```python
from build123d import *

# Parameters (mm, degrees)
SKETCH1_R           = 28
SKETCH1_R_2         = 19.25
BOSS_EXTRUDE1_DEPTH = 2
SKETCH2_R           = 22.15
SKETCH2_R_2         = 19.25
BOSS_EXTRUDE2_DEPTH = 1
SKETCH3_R           = 1.375
CUT_EXTRUDE1_DEPTH  = 4
SKETCH4_W           = 12.894615696
SKETCH4_H           = 54.223512158
CUT_EXTRUDE2_DEPTH  = 4
FILLET1_R           = 10
SKETCH5_R           = 2.35
CUT_EXTRUDE3_DEPTH  = 1.5
CHAMFER2_SIZE       = 0.9
CHAMFER1_SIZE       = 1
CHAMFER3_SIZE       = 1.25


with BuildPart() as part:
    # Sketch1 → Boss-Extrude1 (new body)
    with BuildSketch(Plane.XY):
        Circle(SKETCH1_R)
        Circle(SKETCH1_R_2, mode=Mode.SUBTRACT)
    extrude(amount=BOSS_EXTRUDE1_DEPTH)

    # Sketch2 → Boss-Extrude2 (add)
    with BuildSketch(Plane(origin=(0, 0, 0), x_dir=(-1, 0, 0), z_dir=(0, 0, -1))):
        Circle(SKETCH2_R)
        Circle(SKETCH2_R_2, mode=Mode.SUBTRACT)
    extrude(amount=BOSS_EXTRUDE2_DEPTH)

    # Sketch3 → Cut-Extrude1 (cut, through all)
    with BuildSketch(Plane.XY.offset(2)):
        with Locations((0, 23.75)):
            Circle(SKETCH3_R)
        with Locations((20.56810334, 11.875)):
            Circle(SKETCH3_R)
        with Locations((20.56810334, -11.875)):
            Circle(SKETCH3_R)
        with Locations((0, -23.75)):
            Circle(SKETCH3_R)
        with Locations((-20.56810334, -11.875)):
            Circle(SKETCH3_R)
        with Locations((-20.56810334, 11.875)):
            Circle(SKETCH3_R)
    extrude(amount=-CUT_EXTRUDE1_DEPTH, mode=Mode.SUBTRACT)

    # Sketch4 → Cut-Extrude2 (cut, through all)
    with BuildSketch(Plane.XY.offset(2)):
        with Locations((30.947307848, -0.328141479)):
            Rectangle(SKETCH4_W, SKETCH4_H)
        with Locations((-30.947307848, -0.328141479)):
            Rectangle(SKETCH4_W, SKETCH4_H)
    extrude(amount=-CUT_EXTRUDE2_DEPTH, mode=Mode.SUBTRACT)

    # Fillet1
    fillet1_edges = [part.edges().sort_by_distance(p)[0] for p in [
        (24.5, -13.555441712, 1),
        (24.5, 13.555441712, 1),
        (-24.5, 13.555441712, 1),
        (-24.5, -13.555441712, 1),
    ]]
    fillet(fillet1_edges, radius=FILLET1_R)

    # Sketch5 → Cut-Extrude3 (cut)
    with BuildSketch(Plane.XY.offset(2)):
        with Locations((0, 23.75)):
            Circle(SKETCH5_R)
        with Locations((20.56810334, 11.875)):
            Circle(SKETCH5_R)
        with Locations((-20.56810334, 11.875)):
            Circle(SKETCH5_R)
        with Locations((20.56810334, -11.875)):
            Circle(SKETCH5_R)
        with Locations((0, -23.75)):
            Circle(SKETCH5_R)
        with Locations((-20.56810334, -11.875)):
            Circle(SKETCH5_R)
    extrude(amount=-CUT_EXTRUDE3_DEPTH, mode=Mode.SUBTRACT)

    # Chamfer2
    chamfer2_edges = [part.edges().sort_by_distance(p)[0] for p in [
        (-2.35, 23.75, 0.5),
        (-22.91810334, -11.875, 0.5),
        (-2.35, -23.75, 0.5),
        (18.21810334, -11.875, 0.5),
        (-22.91810334, 11.875, 0.5),
        (18.21810334, 11.875, 0.5),
    ]]
    chamfer(chamfer2_edges, length=CHAMFER2_SIZE)

    # Chamfer1
    chamfer1_edges = [part.edges().sort_by_distance(p)[0] for p in [
        (-19.25, 0, 2),
        (0, 28, 2),
        (24.5, 0, 2),
        (-24.5, 0, 2),
        (0, -28, 2),
        (-24.001461876, 13.783412326, 2),
        (-24.001461876, -13.783412326, 2),
        (24.001461876, -13.783412326, 2),
        (24.001461876, 13.783412326, 2),
    ]]
    chamfer(chamfer1_edges, length=CHAMFER1_SIZE)

    # Chamfer3
    chamfer3_edges = [part.edges().sort_by_distance(p)[0] for p in [
        (19.25, 0, -1),
    ]]
    chamfer(chamfer3_edges, length=CHAMFER3_SIZE)


solid = part.part
```
Work out the finished part from the listing and answer in its coordinate system (mm). A direction names the side the tool comes from. Coordinates: 2 decimals unless noted, no trailing zeros. Use a Markdown table: item, result.
Item 1: For faces 1 (the cylindrical face through (0.367, 27.998, 0.493)), 2 (the cylindrical face through (22.739, -12.775, 1.704)), 3 (the flat face through (-22, 6, 0)), determine the directions among +Z, -Z, +X, -X, +Y, -Y from which every point of the face is accessible in a straight line to the end or side of a thin tool.
Evaluation:
| item | result |
|---|---|
| face 1 | +Z, -Z, +Y |
| face 2 | +Z |
| face 3 | -Z |
Item 2: Given pin 1 Ø1 at (x, z) = (-10, 1.5) entering from -Y; pin 2 Ø3 at (x, y) = (-20.5, -12) entering from +Z; pin 3 Ø4 at (x, y) = (20.57, 11.88) entering from +Z, each flat-ended and moving along its own axis, determine where each tip first touches the part or whether it passes through.
Evaluation:
| item | result |
|---|---|
| pin 1 | stops at y = -26.19 |
| pin 2 | stops at z = 0.69 |
| pin 3 | stops at z = 1.06 |
Item 3: Consider probe 1 along Y at (x, z) = (-1, 0.9); probe 2 along Y at (x, z) = (0, 1.2); probe 3 along X at (y, z) = (-11.5, 0.4). Determine where each line is inside the solid, lowest interval first. Write a range as from..to.
Evaluation:
| item | result |
|---|---|
| probe 1 | y = -27.98..-25.31, -22.19..-19.22, 19.22..22.19, 25.31..27.98 |
| probe 2 | y = -27.8..-25.9, -21.6..-19.45, 19.45..21.6, 25.9..27.8 |
| probe 3 | x = -24.47..-21.89, -19.25..-15.44, 15.44..19.25, 21.89..24.47 |
Item 4: The mould has two halves that part along X. Classify faces 4 (the cylindrical face through (4.802, -21.623, -0.493)), 5 (the cylindrical face through (21.88, 12.29, 0.25)), 6 (the cylindrical face through (-23.988, -13.826, 0.493)), 7 (the cylindrical face through (-19.257, -11.462, 0.254)): +X half, -X half, draft (parallel to the pull), parting line (faces both ways), or undercut.
Evaluation:
| item | result |
|---|---|
| face 4 | parting line |
| face 5 | undercut |
| face 6 | -X half |
| face 7 | undercut |
